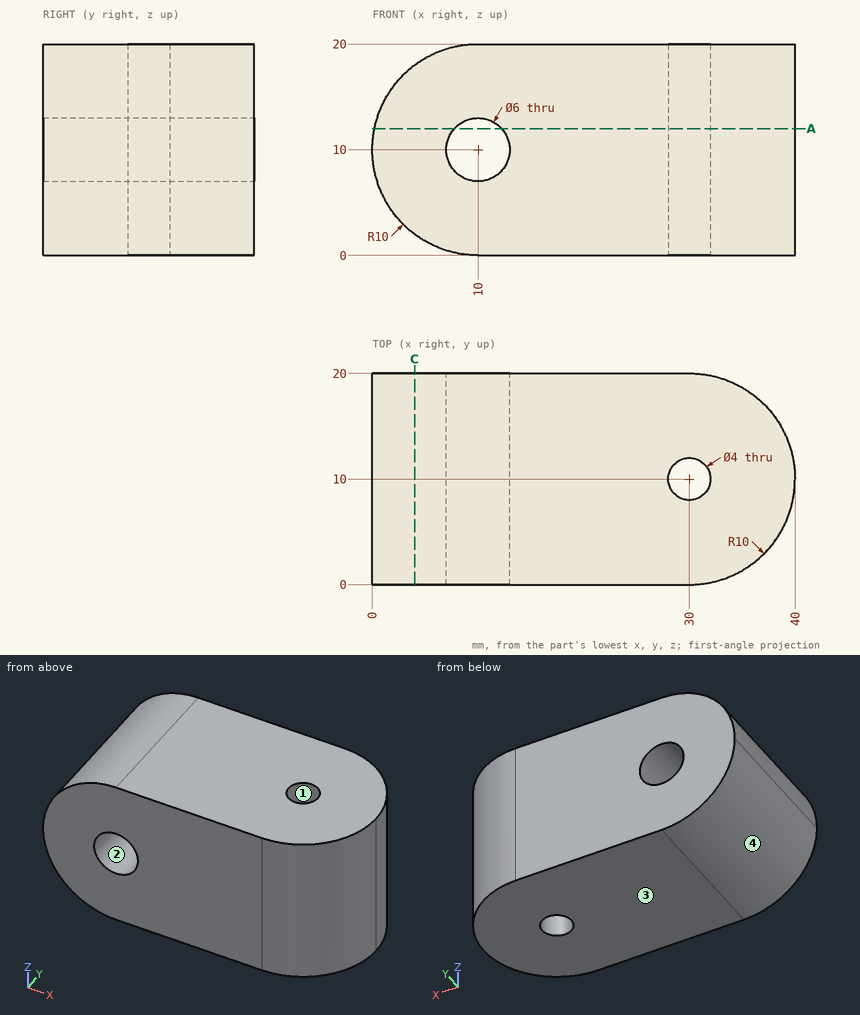
The drawing under review shows one solid part. Ordinate dimensions are in mm from its lowest x, y, z. Coordinates: 2 decimals unless noted, no trailing zeros. Write each loop counter-clockwise with the first axis right and the second up, starting at its lowest first coordinate (ties: lowest second). Pieces come first, ordered by that corner, then holes. Notation, with made-up numbers: (31, 6) - (90, 6) arc R20 cw to (90, 36) - close; hole circle Ø5 at (53, -12). An arc over 180 degrees is marked (long way). Answer in a Markdown table with one row per item. Add a question column.
Q1. For probe 1 along Z at (x, y) = (10, 10.5); probe 2 along X at (y, z) = (3.5, 9.25); probe 3 along X at (y, z) = (7.5, 7.25), list the stretches that pass through material, from the lowest coordinate up.
Q2. We need section C-C, the plane x = 4. State the section outline as (y, z) points, and give its area (3 significant figures).
Q3. For P1, Ø12, axis at y = 6, z = 18, coming from the -X side; P2, Ø1.5, axis at y = 15.5, z = 3, coming from the -X side; P3, Ø6, axis at y = 17, z = 17.5, coming from the +X side; P4, Ø5, axis at x = 10, z = 10, coming from the -Y side, all flat-tipped, find the tip position at first contact; note any pin that passes through.
Q4. Draft analysis for pull direction X (two halves, no side actions). For the marked faces 1, 2, 3 and 4, state which applies: +X half, -X half, draft (parallel to the pull), parting line (faces both ways), or undercut.
Q5. We need section A-A, the plane z = 12. Count the separate pieces of the cut face and the enclosed holes in it, and give its area (3 significant figures).
Answer list:
| question | item | result |
|---|---|---|
| 1 | probe 1 | z = 0 to 7, 13 to 20 |
| 1 | probe 2 | x = 0.03 to 7.1, 12.9 to 37.6 |
| 1 | probe 3 | x = 0.39 to 8.8, 11.2 to 39.68 |
| 2 | outline | (0, 2) - (20, 2) - (20, 18) - (0, 18) - close |
| 2 | area | 320 mm2 |
| 3 | P1 | stops at x = 0.2 |
| 3 | P2 | stops at x = 2.19 |
| 3 | P3 | stops at x = 39.17 |
| 3 | P4 | passes through |
| 4 | face 1 | undercut |
| 4 | face 2 | undercut |
| 4 | face 3 | draft |
| 4 | face 4 | -X half |
| 5 | separate pieces | 2 |
| 5 | enclosed holes | 1 |
| 5 | area | 651 mm2 |
